Could you check a few things on this model? Use its own coordinates, in mm. Face numbers are marked on the shaded views. A direction names the side the tool comes from. Round coordinates to 2 decimals unless told otherwise and drop trailing zeros. Loops run counter-clockwise (first coordinate to the right, second up) from the corner with the lowest first, then second, coordinate; pieces in that order, holes last. Notation, with made-up numbers: (31, 73.25) -> (80, 73.25) arc R37 ccw to (80, 112.25) -> close; hole circle Ø11 at (-39, 87.25). An arc over 180 degrees is marked (long way). Write each question's results on one line, items separated by ' | '.
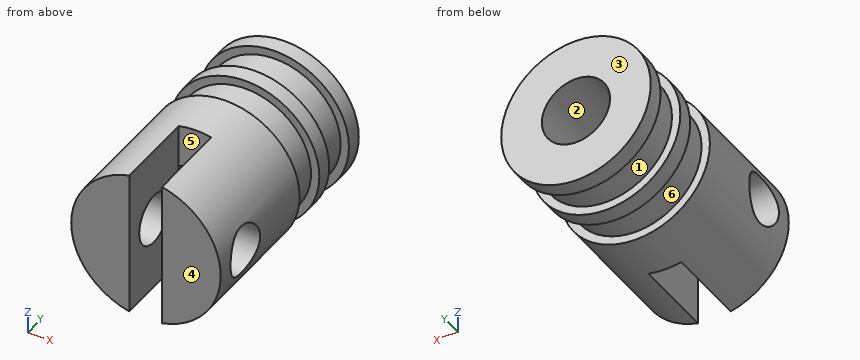
from build123d import *

# Parameters (mm, degrees)
CROQUIS3_W                 = 1.967221418
CROQUIS3_H                 = 9
CORTAR_EXTRUIR1_DEPTH      = 5
CROQUIS4_R                 = 2.05
CORTAR_EXTRUIR2_DEPTH      = 9
CROQUIS7_R                 = 1.5
CORTAR_EXTRUIR3_DEPTH      = 6.467221418
CORTAR_EXTRUIR3_DEPTH_BACK = 4.532778582
ESCALA1_SCALE              = 7


with BuildPart() as part:
    # Croquis2 → Revolución4 (revolve)
    with BuildSketch(Plane.XY):
        Polygon((0, 14), (-4.5, 14), (-4.5, 13), (-4, 13), (-4, 11), (-4.5, 11), (-4.5, 10), (-4, 10), (-4, 8), (-4.5, 8), (-4.5, 0), (0, 0), align=None)
    revolve(axis=Axis((0, 0, 0), (0, 1, 0)))

    # Croquis3 → Cortar-Extruir1 (cut)
    with BuildSketch(Plane.XZ):
        with Locations((-0.016389291, 0)):
            Rectangle(CROQUIS3_W, CROQUIS3_H)
    extrude(amount=-CORTAR_EXTRUIR1_DEPTH, mode=Mode.SUBTRACT)

    # Croquis4 → Cortar-Extruir2 (cut)
    with BuildSketch(Plane(origin=(0, 14, 0), x_dir=(1, 0, 0), z_dir=(0, 1, 0))):
        Circle(CROQUIS4_R)
    extrude(amount=-CORTAR_EXTRUIR2_DEPTH, mode=Mode.SUBTRACT)

    # Croquis7 → Cortar-Extruir3 (cut, two sides)
    with BuildSketch(Plane.ZY.offset(-0.967221418)) as cortar_extruir3_sk:
        with Locations((0, 2.5)):
            Circle(CROQUIS7_R)
    extrude(amount=CORTAR_EXTRUIR3_DEPTH, mode=Mode.SUBTRACT)
    extrude(cortar_extruir3_sk.sketch, amount=-CORTAR_EXTRUIR3_DEPTH_BACK, mode=Mode.SUBTRACT)


with BuildPart() as part_1:
    # Escala1: scaled about (0.00203743, 7.224994078, -4.8862e-05)
    add(part.part.scale(ESCALA1_SCALE).moved(Location((-0.01222458, -43.349964468, 0.000293172))))


solid = part_1.part
1) I need wall thicknesses on line 1 (Y direction, x = -20, z = -23); line 2 (X direction, y = 48.5, z = 0.5); line 3 (Y direction, x = 2, z = -18.5). Which ranges of each line are inside material? Lowest first, please.
Model answer:
line 1: y = -43.35 to 12.65, 26.65 to 33.65, 47.65 to 54.65 | line 2: x = -31.51 to -14.35, 14.33 to 31.48 | line 3: y = -8.35 to 54.65
2) I want a section at C-C, the plane z = -20. Write out the boundary of the cut face in (x, y).
Model answer:
outline: (-24.35, -43.35) -> (-7.01, -43.35) -> (-7.01, -8.35) -> (6.76, -8.35) -> (6.76, -43.35) -> (24.32, -43.35) -> (24.32, 12.65) -> (19.58, 12.65) -> (19.58, 26.65) -> (24.32, 26.65) -> (24.32, 33.65) -> (19.58, 33.65) -> (19.58, 47.65) -> (24.32, 47.65) -> (24.32, 54.65) -> (-24.35, 54.65) -> (-24.35, 47.65) -> (-19.61, 47.65) -> (-19.61, 33.65) -> (-24.35, 33.65) -> (-24.35, 26.65) -> (-19.61, 26.65) -> (-19.61, 12.65) -> (-24.35, 12.65) -> close
3) I'm going to push flat-ended pins straight in: pin 1 (3 mm diameter, centred on y = 0.5, z = 14, fed in from -X); pin 2 (19 mm diameter, centred on x = 2, z = 9, fed in from -Y); pin 3 (3 mm diameter, centred on y = -2.5, z = -24.5, fed in from +X); pin 4 (5 mm diameter, centred on x = -21.5, y = 39, fed in from -Z). Where does each tip first touch, or does it pass through?
Model answer:
pin 1: stops at x = -28.93 | pin 2: stops at y = -43.35 | pin 3: stops at x = 21.51 | pin 4: stops at z = -20.58
4) I want a section at B-B, the plane x = 11. Write out the boundary of the cut face in (y, z), plus the area to 3 significant figures.
Model answer:
outline: (-43.35, -29.51) -> (12.65, -29.51) -> (12.65, -25.74) -> (26.65, -25.74) -> (26.65, -29.51) -> (33.65, -29.51) -> (33.65, -25.74) -> (47.65, -25.74) -> (47.65, -29.51) -> (54.65, -29.51) -> (54.65, -9.2) -> (-8.35, -9.2) -> (-8.35, 9.2) -> (54.65, 9.2) -> (54.65, 29.51) -> (47.65, 29.51) -> (47.65, 25.74) -> (33.65, 25.74) -> (33.65, 29.51) -> (26.65, 29.51) -> (26.65, 25.74) -> (12.65, 25.74) -> (12.65, 29.51) -> (-43.35, 29.51) -> close; hole circle Ø21 at (-25.85, 0) | area: 4,070 mm2
5) I want a section at D-D, the plane y = 16.5. Write out the boundary of the cut face in (x, z), plus the area to 3 significant figures.
Model answer:
outline: circle Ø56 at (-0.01, 0); hole circle Ø28.7 at (-0.01, 0) | area: 1,820 mm2
6) I want a section at A-A, the plane y = -33. Write out the boundary of the cut face in (x, z), plus the area to 3 significant figures.
Model answer:
outline: (-30.56, -7.69) arc R31.5 ccw to (-7.01, -30.71) -> (-7.01, -7.69) -> close; (-30.56, 7.69) -> (-7.01, 7.69) -> (-7.01, 30.71) arc R31.5 ccw to start; (6.76, -30.76) arc R31.5 ccw to (30.53, -7.69) -> (6.76, -7.69) -> close; (6.76, 7.69) -> (30.53, 7.69) arc R31.5 ccw to (6.76, 30.76) -> close | area: 1,510 mm2
7) For the marked faces 4, 5 and 6, which set-ups out of +Z, -Z, +X, -X, +Y, -Y let a thin tool reach every point of the face, with its end or its side?
Model answer:
face 4: +Z, -Z, +X, -X, -Y | face 5: +Z, -Z, -Y | face 6: none
8) If we mould it in two halves opening along X, with no side actions, what happens to the marked faces 1, 2 and 3? For each: released by +X, released by -X, zero draft, split by the parting line, or undercut.
Model answer:
face 1: split by the parting line | face 2: undercut | face 3: zero draft
